Autodesk Inventor part; units mm, degrees
ref_plane "YZ Plane" through (0, 0, 0) normal (1, 0, 0) x (0, 1, 0)
ref_plane "XZ Plane" through (0, 0, 0) normal (0, 1, 0) x (-1, 0, 0)
ref_plane "XY Plane" through (0, 0, 0) normal (0, 0, 1) x (1, 0, 0)
sketch "Sketch1" plane through (0, 0, 0) normal (0, 1, 0) x (-1, 0, 0)
  circle A0 centre (0, 0.2173) radius 16
  point P0 (0, 0)
  dimension "d0" = 32
extrude "Extrusion1" add sketch "Sketch1" along normal blind 1.5
sketch "Sketch2" plane through (0, 1.5, 0.2173) normal (0, 1, 0) x (1, 0, 0)
  circle A0 centre (0, 0.2173) radius 14.5
  dimension "d3" = 29
extrude "Extrusion2" cut sketch "Sketch2" against normal blind 1.5
sketch "Sketch3" plane through (0, 1.5, 0.2173) normal (0, 1, 0) x (1, 0, 0)
  line L0 (-1, -17.209) -> (1, -17.209)
  line L1 (1, -17.209) -> (1, -13.4717)
  line L2 (1, -13.4717) -> (-1, -13.4717)
  line L3 (-1, -13.4717) -> (-1, -17.209)
  line L4 (-1, -17.209) -> (1, -13.4717) construction
  line L5 (1, -17.209) -> (-1, -13.4717) construction
  point P0 (0, 0.2173)
  point P1 (0, -15.3403)
  dimension "d6" = 2
extrude "Extrusion3" cut sketch "Sketch3" against normal blind 1.5
properties part number "piston compression ring"
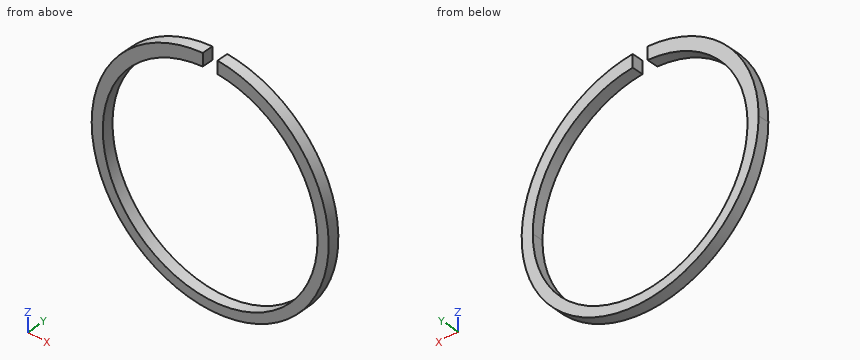
Here's how the part is built. I have some questions about the finished solid (model axes, mm). Coordinates: 2 decimals unless noted, no trailing zeros. Loops run counter-clockwise (first coordinate to the right, second up) from the corner with the lowest first, then second, coordinate; pieces in that order, holes last. Notation, with made-up numbers: (-15.75, 77.5) -> (-11.75, 77.5) arc R20 ccw to (-11.75, 82.5) -> close; hole circle Ø2 at (17.25, -25.75). An arc over 180 degrees is marked (long way). Return JSON: item names as keys, results as strings.
1) If we section it at D-D, the plane x = 0: Write out the boundary of the cut face in (y, z).
Results below:
{"outline": "(0, -15.78) -> (1.5, -15.78) -> (1.5, -14.5) -> (0, -14.5) -> close"}
2) Will these pins go through, and if not, where does the flat tip stop? pin 1 (4 mm diameter, centred on x = -6, z = -9, fed in from -Y); pin 2 (0.8 mm diameter, centred on y = 1, z = 15, fed in from -X).
Results below:
{"pin 1": "through", "pin 2": "x = -7.01"}
3) If we section it at C-C, the plane y = 0.95: Write out the boundary of the cut face in (x, z).
Results below:
{"outline": "(-1, 14.47) -> (-1, 16.19) arc R16 ccw (long way) to (1, 16.19) -> (1, 14.47) arc R14.5 cw (long way) to start"}
4) If we section it at A-A, the plane x = -6: Write out the boundary of the cut face in (y, z).
Results below:
{"outline": "(0, -14.62) -> (1.5, -14.62) -> (1.5, -13.2) -> (0, -13.2) -> close; (0, 13.2) -> (1.5, 13.2) -> (1.5, 15.05) -> (0, 15.05) -> close"}
5) I need wall thicknesses on line 1 (X direction, y = 0.3, z = 0); line 2 (Z direction, x = 0, y = 1.1); line 3 (X direction, y = 0.1, z = -4.5). Which ranges of each line are inside material? Lowest first, please. Write a range as from..to.
Results below:
{"line 1": "-16..-14.5, 14.5..16", "line 2": "-15.78..-14.5", "line 3": "-15.29..-13.78, 13.78..15.29"}
6) If we section it at B-B, the plane z = 5: Write out the boundary of the cut face in (x, y).
Results below:
{"outline": "(-15.27, 0) -> (-13.61, 0) -> (-13.61, 1.5) -> (-15.27, 1.5) -> close; (13.61, 0) -> (15.27, 0) -> (15.27, 1.5) -> (13.61, 1.5) -> close"}
